```python
from build123d import *

# Parameters (mm, degrees)
FILLET_R     = 0.2
POCKET_DEPTH = 0.5
FILLET001_R  = 0.05


with BuildPart() as part:
    # Sketch → Revolution (revolve)
    with BuildSketch(Plane.XY):
        Polygon((0, 0), (0, 11.3), (1.55, 11.3), (1.55, 10), (1, 10), (1, 0), align=None)
    revolve(axis=Axis((0, 0, 0), (0, 1, 0)))

    # Fillet
    fillet_edges = [part.edges().sort_by_distance(p)[0] for p in [
        (-1.55, 11.3, 0),
        (-1.55, 10, 0),
    ]]
    fillet(fillet_edges, radius=FILLET_R)

    # Sketch001 (on Face1 of Fillet) → Pocket (cut)
    with BuildSketch(Plane(origin=(0, 11.3, 0), x_dir=(-1, 0, 0), z_dir=(0, 1, 0))):
        Polygon((0, 1), (0.3, 1), (0.3, 0.3), (1, 0.3), (1, -0.3), (0.3, -0.3), (0.3, -1), (0, -1), align=None)
    pocket = extrude(amount=-POCKET_DEPTH, mode=Mode.SUBTRACT)

    # Mirrored: Pocket across Sketch001 V_Axis
    add(pocket.mirror(Plane(origin=(0, 11.3, 0), x_dir=(0, 1, 0), z_dir=(-1, 0, 0))), mode=Mode.SUBTRACT)

    # Fillet001
    fillet001_edges = [part.edges().sort_by_distance(p)[0] for p in [
        (-0.65, 11.3, 0.3),
        (-1, 11.3, 0),
        (-0.65, 11.3, -0.3),
        (-0.3, 11.3, -0.65),
        (-0.15, 11.3, -1),
        (0.15, 11.3, -1),
        (0.3, 11.3, -0.65),
        (0.65, 11.3, -0.3),
        (0.65, 11.3, 0.3),
        (1, 11.3, 0),
        (0.3, 11.3, 0.65),
        (-0.3, 11.3, 0.65),
        (-0.15, 11.3, 1),
        (0.15, 11.3, 1),
    ]]
    fillet(fillet001_edges, radius=FILLET001_R)


solid = part.part
```
Source: CAD feature listing. Evaluate the final solid. Frame: model axes, mm. Coordinates: 2 decimals unless noted, no trailing zeros. Write each loop counter-clockwise with the first axis right and the second up, starting at its lowest first coordinate (ties: lowest second). Pieces come first, ordered by that corner, then holes. Notation, with made-up numbers: (-29.75, 36) -> (26.25, 36) arc R31 cw to (26.25, 67) -> close; hole circle Ø10 at (80, -25.5). An arc over 180 degrees is marked (long way). Return JSON: item names as keys, results as strings. Group by question number.
1) Section query B-B, the plane z = 0. Return loops of the section in (x, y).
2) Section query C-C, the plane y = 3. Return loops of the section in (x, z).
3) Section query A-A, the plane x = 0. Return loops of the section in (y, z).
4) Ray query, line 1 along Y through (x, z) = (-0.15, -1.15); line 2 along X through (y, z) = (4.5, 0); line 3 along Z through (x, y) = (0.7, 3). Return the intervals inside material, ascending.
5) Mould query, pull axis X, two halves, no side actions, for faces 1 (the face through (0, 0, 0)), 2 (the face through (0, 10.8, 0)), 3 (the face through (0, 5, 1)). Classes: +X half, -X half, draft (parallel to the pull), parting line (faces both ways), or undercut.
6) Contact query for flat-ended pins moving along their axis: P1, Ø0.5, axis at y = 11, z = -0.5, coming from the -X side; P2, Ø0.5, axis at x = 0.5, y = 11, coming from the -Z side; P3, Ø1.5, axis at x = -0.5, y = 6, coming from the +Z side. Output: stop coordinate, or through.
From the geometry:
{
 "1": {"outline": "(-1.55, 10.2) arc R0.2 ccw to (-1.35, 10) -> (-1, 10) -> (-1, 0) -> (1, 0) -> (1, 10) -> (1.35, 10) arc R0.2 ccw to (1.55, 10.2) -> (1.55, 11.1) arc R0.2 ccw to (1.35, 11.3) -> (1.05, 11.3) arc R0.05 ccw to (1, 11.25) -> (1, 10.8) -> (-1, 10.8) -> (-1, 11.25) arc R0.05 ccw to (-1.05, 11.3) -> (-1.35, 11.3) arc R0.2 ccw to (-1.55, 11.1) -> close"},
 "2": {"outline": "circle Ø2 at (0, 0)"},
 "3": {"outline": "(0, -1) -> (10, -1) -> (10, -1.35) arc R0.2 ccw to (10.2, -1.55) -> (11.1, -1.55) arc R0.2 ccw to (11.3, -1.35) -> (11.3, -1.05) arc R0.05 ccw to (11.25, -1) -> (10.8, -1) -> (10.8, 1) -> (11.25, 1) arc R0.05 ccw to (11.3, 1.05) -> (11.3, 1.35) arc R0.2 ccw to (11.1, 1.55) -> (10.2, 1.55) arc R0.2 ccw to (10, 1.35) -> (10, 1) -> (0, 1) -> close"},
 "4": {"line 1": "10 to 11.3", "line 2": "-1 to 1", "line 3": "-0.71 to 0.71"},
 "5": {"face 1": "draft", "face 2": "undercut", "face 3": "parting line"},
 "6": {"P1": "x = -1.53", "P2": "z = -1.53", "P3": "z = 1"}
}
